Build history of the part. All positions in model axes, mm. A direction names the side the tool comes from. Give positions to 0.01 mm unless a question says otherwise; leave off trailing zeros. Write each loop counter-clockwise with the first axis right and the second up, starting at its lowest first coordinate (ties: lowest second). Pieces come first, ordered by that corner, then holes.
from build123d import *

# Parameters (mm, degrees)
SKETCH1_W           = 21
SKETCH1_H           = 5.5
BOSS_EXTRUDE1_DEPTH = 8
SKETCH2_W           = 21
SKETCH2_H           = 5.1
CUT_EXTRUDE1_DEPTH  = 5.5
SKETCH4_W           = 18
SKETCH4_H           = 3
CUT_EXTRUDE2_DEPTH  = 5.5
SKETCH5_R           = 1.5
CUT_EXTRUDE3_DEPTH  = 10.5


with BuildPart() as part:
    # Sketch1 → Boss-Extrude1 (new body)
    with BuildSketch(Plane(origin=(0, 0, 0), x_dir=(1, 0, 0), z_dir=(0, 1, 0))):
        Polygon((-20, 20), (-20, 12), (-10.5, 12), (-10.5, 17.5), (10.5, 17.5), (10.5, 12), (20, 12), (20, 20), align=None)
        with Locations((0, 14.75)):
            Rectangle(SKETCH1_W, SKETCH1_H)
    extrude(amount=BOSS_EXTRUDE1_DEPTH)

    # Sketch2 → Cut-Extrude1 (cut)
    with BuildSketch(Plane.XY.offset(-12)):
        with Locations((0, 4)):
            Rectangle(SKETCH2_W, SKETCH2_H)
    extrude(amount=-CUT_EXTRUDE1_DEPTH, mode=Mode.SUBTRACT)

    # Sketch4 → Cut-Extrude2 (cut)
    with BuildSketch(Plane.XY.offset(-17.5)):
        with Locations((0, 4)):
            Rectangle(SKETCH4_W, SKETCH4_H)
    extrude(amount=-CUT_EXTRUDE2_DEPTH, mode=Mode.SUBTRACT)

    # Sketch5 → Cut-Extrude3 (cut)
    with BuildSketch(Plane(origin=(0, 0, -20), x_dir=(-1, 0, 0), z_dir=(0, 0, -1))):
        with Locations((-16, 4)):
            Circle(SKETCH5_R)
        with Locations((16, 4)):
            Circle(SKETCH5_R)
    extrude(amount=-CUT_EXTRUDE3_DEPTH, mode=Mode.SUBTRACT)


solid = part.part
1. 3-axis set-ups, long thin cutter, end or side, ignore diameter. For faces 1 (the face through (9, 4, -19)), 2 (the face through (20, 4, -16)), 3 (the face through (0, 6.55, -15)): which of +Z, -Z, +X, -X, +Y, -Y reach the whole face in a straight line?
2. Drill centre lines: line 1 along Y through (x, z) = (6, -16.25); line 2 along Y through (x, z) = (-16, -16); line 3 along X through (y, z) = (3.5, -18.25). Where is each one in solid material? Low to high.
3. Saw through at A-A on x = -1. Give the cut face in (y, z).
4. Saw through at D-D on x = 16. Give the cut face in (y, z), plus the area to 3 significant figures.
5. Mould opens along X. For faces 4 (the face through (0, 6, -20)), 5 (the face through (-14.5, 4.07, -16.06)), 6 (the face through (-20, 4, -16)), 7 (the face through (-10.5, 4, -15)) say: pulls with the +X half, pulls with the -X half, needs draft (parallel to the pull), parting line crosses it, or undercut.
6. Saw through at B-B on z = -13.75. Give the cut face in (x, y), plus the area to 3 significant figures.
7. Saw through at C-C on y = 4. Give the cut face in (x, z).
Outcome:
1. face 1: +Z, -Z
1. face 2: +Z, -Z, +X, +Y, -Y
1. face 3: +Z
2. line 1: y = 0 to 1.45, 6.55 to 8
2. line 2: y = 0 to 2.5, 5.5 to 8
2. line 3: x = -20 to -17.41, -14.59 to -9, 9 to 14.59, 17.41 to 20
3. outline: (0, -20) - (2.5, -20) - (2.5, -17.5) - (1.45, -17.5) - (1.45, -12) - (0, -12) - close; (5.5, -20) - (8, -20) - (8, -12) - (6.55, -12) - (6.55, -17.5) - (5.5, -17.5) - close
4. outline: (0, -20) - (2.5, -20) - (2.5, -12) - (0, -12) - close; (5.5, -20) - (8, -20) - (8, -12) - (5.5, -12) - close
4. area: 40.0 mm2
5. face 4: needs draft
5. face 5: undercut
5. face 6: pulls with the -X half
5. face 7: undercut
6. outline: (-20, 0) - (20, 0) - (20, 8) - (-20, 8) - close; hole circle Ø3 at (-16, 4); hole (-10.5, 1.45) - (10.5, 1.45) - (10.5, 6.55) - (-10.5, 6.55) - close; hole circle Ø3 at (16, 4)
6. area: 199 mm2
7. outline: (-20, -20) - (-17.5, -20) - (-17.5, -12) - (-20, -12) - close; (-14.5, -20) - (-9, -20) - (-9, -17.5) - (-10.5, -17.5) - (-10.5, -12) - (-14.5, -12) - close; (9, -20) - (14.5, -20) - (14.5, -12) - (10.5, -12) - (10.5, -17.5) - (9, -17.5) - close; (17.5, -20) - (20, -20) - (20, -12) - (17.5, -12) - close
